Geometry: final body of the model. Coordinates: model frame, mm. Give positions to 0.01 mm unless a question says otherwise; leave off trailing zeros. Order: outer loops, then holes, each group sorted by start corner. A loop starts at its lowest first (then second) coordinate and runs counter-clockwise, first axis right, second up. Notation, with made-up numbers: (-3, 52) - (30, 52) arc R19 ccw to (30, 72) - close; hole circle Ø10 at (71, 56). An arc over 180 degrees is marked (long way). Put each result on its own line as item: value. Start each with the question number.
1. Section B-B on x = -8. Return the cut outline in (y, z), plus the area to 3 significant figures.
2. Ray query, line 1 along X through (y, z) = (1.35, -50); line 2 along X through (y, z) = (-0.2, 37); line 3 along Z through (x, y) = (17, 1.8). Return the intervals inside material, ascending. Write a range as from..to.
3. Section C-C on y = -1.35. Count the separate pieces of the cut face and the enclosed holes in it, plus the area to 3 significant figures.
4. Section A-A on x = -116.5. Return the cut outline in (y, z).
from build123d import *

# Parameters (mm, degrees)
SKETCH1_W           = 300
SKETCH1_H           = 140
BOSS_EXTRUDE1_DEPTH = 2
CUT_EXTRUDE1_REACH  = 167.578
CUT_EXTRUDE2_REACH  = 167.578
SKETCH3_W           = 30
SKETCH3_H           = 4
FILLET1_R           = 6
SKETCH4_W           = 10
SKETCH4_H           = 4
CUT_EXTRUDE3_DEPTH  = 166.577776287
SKETCH5_W           = 4
SKETCH5_H           = 10
CUT_EXTRUDE4_DEPTH  = 166.577776287
SKETCH6_W           = 18
SKETCH6_H           = 4
CUT_EXTRUDE5_DEPTH  = 166.577776287
SKETCH7_W           = 20
SKETCH7_H           = 4
SKETCH7_W_2         = 4
SKETCH7_H_2         = 10
CUT_EXTRUDE6_DEPTH  = 166.577776287


with BuildPart() as part:
    # Sketch1 → Boss-Extrude1 (new, symmetric)
    with BuildSketch(Plane(origin=(0, 0, 0), x_dir=(1, 0, 0), z_dir=(0, 1, 0))):
        Rectangle(SKETCH1_W, SKETCH1_H)
    extrude(amount=BOSS_EXTRUDE1_DEPTH, both=True)

    # Sketch2 → Cut-Extrude1 (cut, up to next)
    with BuildSketch(Plane(origin=(0, 2, 0), x_dir=(1, 0, 0), z_dir=(0, 1, 0)), mode=Mode.PRIVATE) as cut_extrude1_sk1:
        with BuildLine():
            Line((-107, 60), (-107, 50))
            ThreePointArc((-107, 50), (-110, 47), (-113, 50))
            Line((-113, 50), (-113, 60))
            ThreePointArc((-113, 60), (-110, 63), (-107, 60))
        make_face()
    cut_extrude1_tool1 = extrude(cut_extrude1_sk1.sketch, amount=-CUT_EXTRUDE1_REACH, mode=Mode.PRIVATE) & part.part
    # Sketch2 → Cut-Extrude1 (cut, up to next)
    with BuildSketch(Plane(origin=(0, 2, 0), x_dir=(1, 0, 0), z_dir=(0, 1, 0)), mode=Mode.PRIVATE) as cut_extrude1_sk2:
        with BuildLine():
            Line((107, 60), (107, 50))
            ThreePointArc((107, 50), (110, 47), (113, 50))
            Line((113, 50), (113, 60))
            ThreePointArc((113, 60), (110, 63), (107, 60))
        make_face()
    cut_extrude1_tool2 = extrude(cut_extrude1_sk2.sketch, amount=-CUT_EXTRUDE1_REACH, mode=Mode.PRIVATE) & part.part
    # Sketch2 → Cut-Extrude1 (cut, up to next)
    with BuildSketch(Plane(origin=(0, 2, 0), x_dir=(1, 0, 0), z_dir=(0, 1, 0)), mode=Mode.PRIVATE) as cut_extrude1_sk3:
        with BuildLine():
            Line((107, -60), (107, -50))
            ThreePointArc((107, -50), (110, -47), (113, -50))
            Line((113, -50), (113, -60))
            ThreePointArc((113, -60), (110, -63), (107, -60))
        make_face()
    cut_extrude1_tool3 = extrude(cut_extrude1_sk3.sketch, amount=-CUT_EXTRUDE1_REACH, mode=Mode.PRIVATE) & part.part
    # Sketch2 → Cut-Extrude1 (cut, up to next)
    with BuildSketch(Plane(origin=(0, 2, 0), x_dir=(1, 0, 0), z_dir=(0, 1, 0)), mode=Mode.PRIVATE) as cut_extrude1_sk4:
        with BuildLine():
            Line((-107, -60), (-107, -50))
            ThreePointArc((-107, -50), (-110, -47), (-113, -50))
            Line((-113, -50), (-113, -60))
            ThreePointArc((-113, -60), (-110, -63), (-107, -60))
        make_face()
    cut_extrude1_tool4 = extrude(cut_extrude1_sk4.sketch, amount=-CUT_EXTRUDE1_REACH, mode=Mode.PRIVATE) & part.part
    add(cut_extrude1_tool1.solids().sort_by_distance((-110, 2, -55))[0], mode=Mode.SUBTRACT)
    add(cut_extrude1_tool2.solids().sort_by_distance((110, 2, -55))[0], mode=Mode.SUBTRACT)
    add(cut_extrude1_tool3.solids().sort_by_distance((110, 2, 55))[0], mode=Mode.SUBTRACT)
    add(cut_extrude1_tool4.solids().sort_by_distance((-110, 2, 55))[0], mode=Mode.SUBTRACT)

    # Sketch3 → Cut-Extrude2 (cut, up to next)
    with BuildSketch(Plane(origin=(0, 2, 0), x_dir=(1, 0, 0), z_dir=(0, 1, 0)), mode=Mode.PRIVATE) as cut_extrude2_sk1:
        with Locations((-60, 6)):
            Rectangle(SKETCH3_W, SKETCH3_H)
    cut_extrude2_tool1 = extrude(cut_extrude2_sk1.sketch, amount=-CUT_EXTRUDE2_REACH, mode=Mode.PRIVATE) & part.part
    # Sketch3 → Cut-Extrude2 (cut, up to next)
    with BuildSketch(Plane(origin=(0, 2, 0), x_dir=(1, 0, 0), z_dir=(0, 1, 0)), mode=Mode.PRIVATE) as cut_extrude2_sk2:
        with Locations((-120, 6)):
            Rectangle(SKETCH3_W, SKETCH3_H)
    cut_extrude2_tool2 = extrude(cut_extrude2_sk2.sketch, amount=-CUT_EXTRUDE2_REACH, mode=Mode.PRIVATE) & part.part
    # Sketch3 → Cut-Extrude2 (cut, up to next)
    with BuildSketch(Plane(origin=(0, 2, 0), x_dir=(1, 0, 0), z_dir=(0, 1, 0)), mode=Mode.PRIVATE) as cut_extrude2_sk3:
        with Locations((0, 6)):
            Rectangle(SKETCH3_W, SKETCH3_H)
    cut_extrude2_tool3 = extrude(cut_extrude2_sk3.sketch, amount=-CUT_EXTRUDE2_REACH, mode=Mode.PRIVATE) & part.part
    # Sketch3 → Cut-Extrude2 (cut, up to next)
    with BuildSketch(Plane(origin=(0, 2, 0), x_dir=(1, 0, 0), z_dir=(0, 1, 0)), mode=Mode.PRIVATE) as cut_extrude2_sk4:
        with Locations((60, 6)):
            Rectangle(SKETCH3_W, SKETCH3_H)
    cut_extrude2_tool4 = extrude(cut_extrude2_sk4.sketch, amount=-CUT_EXTRUDE2_REACH, mode=Mode.PRIVATE) & part.part
    # Sketch3 → Cut-Extrude2 (cut, up to next)
    with BuildSketch(Plane(origin=(0, 2, 0), x_dir=(1, 0, 0), z_dir=(0, 1, 0)), mode=Mode.PRIVATE) as cut_extrude2_sk5:
        with Locations((120, 6)):
            Rectangle(SKETCH3_W, SKETCH3_H)
    cut_extrude2_tool5 = extrude(cut_extrude2_sk5.sketch, amount=-CUT_EXTRUDE2_REACH, mode=Mode.PRIVATE) & part.part
    # Sketch3 → Cut-Extrude2 (cut, up to next)
    with BuildSketch(Plane(origin=(0, 2, 0), x_dir=(1, 0, 0), z_dir=(0, 1, 0)), mode=Mode.PRIVATE) as cut_extrude2_sk6:
        with Locations((120, -6)):
            Rectangle(SKETCH3_W, SKETCH3_H)
    cut_extrude2_tool6 = extrude(cut_extrude2_sk6.sketch, amount=-CUT_EXTRUDE2_REACH, mode=Mode.PRIVATE) & part.part
    # Sketch3 → Cut-Extrude2 (cut, up to next)
    with BuildSketch(Plane(origin=(0, 2, 0), x_dir=(1, 0, 0), z_dir=(0, 1, 0)), mode=Mode.PRIVATE) as cut_extrude2_sk7:
        with Locations((60, -6)):
            Rectangle(SKETCH3_W, SKETCH3_H)
    cut_extrude2_tool7 = extrude(cut_extrude2_sk7.sketch, amount=-CUT_EXTRUDE2_REACH, mode=Mode.PRIVATE) & part.part
    # Sketch3 → Cut-Extrude2 (cut, up to next)
    with BuildSketch(Plane(origin=(0, 2, 0), x_dir=(1, 0, 0), z_dir=(0, 1, 0)), mode=Mode.PRIVATE) as cut_extrude2_sk8:
        with Locations((0, -6)):
            Rectangle(SKETCH3_W, SKETCH3_H)
    cut_extrude2_tool8 = extrude(cut_extrude2_sk8.sketch, amount=-CUT_EXTRUDE2_REACH, mode=Mode.PRIVATE) & part.part
    # Sketch3 → Cut-Extrude2 (cut, up to next)
    with BuildSketch(Plane(origin=(0, 2, 0), x_dir=(1, 0, 0), z_dir=(0, 1, 0)), mode=Mode.PRIVATE) as cut_extrude2_sk9:
        with Locations((-60, -6)):
            Rectangle(SKETCH3_W, SKETCH3_H)
    cut_extrude2_tool9 = extrude(cut_extrude2_sk9.sketch, amount=-CUT_EXTRUDE2_REACH, mode=Mode.PRIVATE) & part.part
    # Sketch3 → Cut-Extrude2 (cut, up to next)
    with BuildSketch(Plane(origin=(0, 2, 0), x_dir=(1, 0, 0), z_dir=(0, 1, 0)), mode=Mode.PRIVATE) as cut_extrude2_sk10:
        with Locations((-120, -6)):
            Rectangle(SKETCH3_W, SKETCH3_H)
    cut_extrude2_tool10 = extrude(cut_extrude2_sk10.sketch, amount=-CUT_EXTRUDE2_REACH, mode=Mode.PRIVATE) & part.part
    add(cut_extrude2_tool1.solids().sort_by_distance((-60, 2, -6))[0], mode=Mode.SUBTRACT)
    add(cut_extrude2_tool2.solids().sort_by_distance((-120, 2, -6))[0], mode=Mode.SUBTRACT)
    add(cut_extrude2_tool3.solids().sort_by_distance((0, 2, -6))[0], mode=Mode.SUBTRACT)
    add(cut_extrude2_tool4.solids().sort_by_distance((60, 2, -6))[0], mode=Mode.SUBTRACT)
    add(cut_extrude2_tool5.solids().sort_by_distance((120, 2, -6))[0], mode=Mode.SUBTRACT)
    add(cut_extrude2_tool6.solids().sort_by_distance((120, 2, 6))[0], mode=Mode.SUBTRACT)
    add(cut_extrude2_tool7.solids().sort_by_distance((60, 2, 6))[0], mode=Mode.SUBTRACT)
    add(cut_extrude2_tool8.solids().sort_by_distance((0, 2, 6))[0], mode=Mode.SUBTRACT)
    add(cut_extrude2_tool9.solids().sort_by_distance((-60, 2, 6))[0], mode=Mode.SUBTRACT)
    add(cut_extrude2_tool10.solids().sort_by_distance((-120, 2, 6))[0], mode=Mode.SUBTRACT)

    # Fillet1
    fillet1_edges = [part.edges().sort_by_distance(p)[0] for p in [
        (150, 0, 70),
        (-150, 0, 70),
        (-150, 0, -70),
        (150, 0, -70),
    ]]
    fillet(fillet1_edges, radius=FILLET1_R)

    # Sketch4 → Cut-Extrude3 (cut, through all)
    with BuildSketch(Plane(origin=(0, 2, 0), x_dir=(1, 0, 0), z_dir=(0, 1, 0))):
        with Locations((20, 30)):
            Rectangle(SKETCH4_W, SKETCH4_H)
        with Locations((-10, 30)):
            Rectangle(SKETCH4_W, SKETCH4_H)
    cut_extrude3 = extrude(amount=-CUT_EXTRUDE3_DEPTH, mode=Mode.SUBTRACT)

    # Sketch5 → Cut-Extrude4 (cut, through all)
    with BuildSketch(Plane(origin=(0, 2, 0), x_dir=(1, 0, 0), z_dir=(0, 1, 0))):
        with Locations((23, 42)):
            Rectangle(SKETCH5_W, SKETCH5_H)
        with Locations((-13, 42)):
            Rectangle(SKETCH5_W, SKETCH5_H)
        with Locations((-13, 62)):
            Rectangle(SKETCH5_W, SKETCH5_H)
        with Locations((23, 62)):
            Rectangle(SKETCH5_W, SKETCH5_H)
    extrude(amount=-CUT_EXTRUDE4_DEPTH, mode=Mode.SUBTRACT)

    # Sketch6 → Cut-Extrude5 (cut, through all)
    with BuildSketch(Plane(origin=(0, 2, 0), x_dir=(1, 0, 0), z_dir=(0, 1, 0))):
        with Locations((-42, 30)):
            Rectangle(SKETCH6_W, SKETCH6_H)
        with Locations((-78, 30)):
            Rectangle(SKETCH6_W, SKETCH6_H)
    cut_extrude5 = extrude(amount=-CUT_EXTRUDE5_DEPTH, mode=Mode.SUBTRACT)

    # Mirror1: Cut-Extrude3, Cut-Extrude5 across plane
    add(cut_extrude3.mirror(Plane.XY), mode=Mode.SUBTRACT)
    add(cut_extrude5.mirror(Plane.XY), mode=Mode.SUBTRACT)

    # Sketch7 → Cut-Extrude6 (cut, through all)
    with BuildSketch(Plane(origin=(0, 2, 0), x_dir=(1, 0, 0), z_dir=(0, 1, 0))):
        with Locations((67, 37.5)):
            Rectangle(SKETCH7_W, SKETCH7_H)
        with Locations((102.5, 37.5)):
            Rectangle(SKETCH7_W, SKETCH7_H)
        with Locations((138, 37.5)):
            Rectangle(SKETCH7_W, SKETCH7_H)
        with Locations((67, -37.5)):
            Rectangle(SKETCH7_W, SKETCH7_H)
        with Locations((102.5, -37.5)):
            Rectangle(SKETCH7_W, SKETCH7_H)
        with Locations((138, -37.5)):
            Rectangle(SKETCH7_W, SKETCH7_H)
        with Locations((53, 42.5)):
            Rectangle(SKETCH7_W_2, SKETCH7_H_2)
        with Locations((53, -42.5)):
            Rectangle(SKETCH7_W_2, SKETCH7_H_2)
    extrude(amount=-CUT_EXTRUDE6_DEPTH, mode=Mode.SUBTRACT)


solid = part.part
Resolved:
1. outline: (-2, -70) - (2, -70) - (2, -32) - (-2, -32) - close; (-2, -28) - (2, -28) - (2, -8) - (-2, -8) - close; (-2, -4) - (2, -4) - (2, 4) - (-2, 4) - close; (-2, 8) - (2, 8) - (2, 28) - (-2, 28) - close; (-2, 32) - (2, 32) - (2, 70) - (-2, 70) - close
1. area: 496 mm^2
2. line 1: -150..-113, -107..107, 113..150
2. line 2: -150..57, 77..92.5, 112.5..128, 148..150
2. line 3: -70..-32, -28..28, 32..70
3. separate pieces: 1
3. enclosed holes: 34
3. area: 39,200 mm^2
4. outline: (-2, -70) - (2, -70) - (2, -8) - (-2, -8) - close; (-2, -4) - (2, -4) - (2, 4) - (-2, 4) - close; (-2, 8) - (2, 8) - (2, 70) - (-2, 70) - close
